Model file for the job. Use its own axes, mm. Face numbers are marked on the shaded views. A direction names the side the tool comes from. Give positions to 0.01 mm unless a question says otherwise; leave off trailing zeros. Write each loop counter-clockwise with the first axis right and the second up, starting at its lowest first coordinate (ties: lowest second). Pieces come first, ordered by that corner, then holes.
```python
from build123d import *

# Parameters (mm, degrees)
F0_W     = 30
F0_H     = 50
F1_DEPTH = 10
F2_R     = 10
F3_DEPTH = 7
F4_R     = 5
F5_R     = 5
F6_R     = 5
F7_R     = 5


with BuildPart() as f1:
    # F0 (on Front) → F1 (new body)
    with BuildSketch(Plane.XZ):
        Rectangle(F0_W, F0_H)
    extrude(amount=-F1_DEPTH)

    # F2 (on face) → F3 (join)
    with BuildSketch(Plane.XZ):
        Circle(F2_R)
    extrude(amount=F3_DEPTH)

    # F4
    f4_edges = [f1.edges().sort_by_distance(p)[0] for p in [
        (15, 5, 25),
    ]]
    fillet(f4_edges, radius=F4_R)

    # F5
    f5_edges = [f1.edges().sort_by_distance(p)[0] for p in [
        (-15, 5, 25),
    ]]
    fillet(f5_edges, radius=F5_R)

    # F6
    f6_edges = [f1.edges().sort_by_distance(p)[0] for p in [
        (15, 5, -25),
    ]]
    fillet(f6_edges, radius=F6_R)

    # F7
    f7_edges = [f1.edges().sort_by_distance(p)[0] for p in [
        (-15, 5, -25),
    ]]
    fillet(f7_edges, radius=F7_R)


solid = f1.part
```
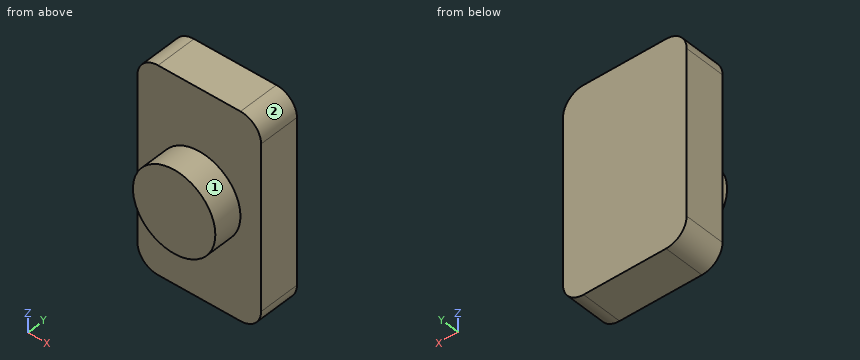
1. Slice it at A-A, the plane x = 0. Write the cut outline in (y, z), and give its area (3 significant figures).
Calculated:
outline: (-7, -10) - (0, -10) - (0, -25) - (10, -25) - (10, 25) - (0, 25) - (0, 10) - (-7, 10) - close
area: 640 mm2
2. Slice it at D-D, the plane x = -10.5. Write the cut outline in (y, z).
Calculated:
outline: (0, -24.97) - (10, -24.97) - (10, 24.97) - (0, 24.97) - close
3. Probe probe 1 along Y at (x, z) = (-9, -23); probe 2 along X at (y, z) = (-4.25, -1.5); probe 3 along Z at (x, y) = (8.75, -1.75). List the from-to ranges inside material, lowest first.
Calculated:
probe 1: y = 0 to 10
probe 2: x = -9.89 to 9.89
probe 3: z = -4.84 to 4.84
4. Slice it at B-B, the plane z = 0. Write the cut outline in (x, y).
Calculated:
outline: (-15, 0) - (-10, 0) - (-10, -7) - (10, -7) - (10, 0) - (15, 0) - (15, 10) - (-15, 10) - close
5. Pin check, flat tips, straight feed: P1, Ø4, axis at x = 10, z = -3.5, coming from the -Y side; P2, Ø1, axis at y = -3.5, z = -11.5, coming from the +X side; P3, Ø1.5, axis at y = -5, z = 7, coming from the +X side. Stop position of each tip, or through.
Calculated:
P1: stops at y = -7
P2: passes through
P3: stops at x = 7.81
6. Which spindle directions (+Z, -Z, +X, -X, +Y, -Y) get a long thin tool onto all of the face, cutting with end or side? Do the marked faces 1 and 2. Say none if no direction does.
Calculated:
face 1: -Y
face 2: +Z, +X, +Y, -Y
7. Slice it at C-C, the plane z = 18.5. Write the cut outline in (x, y), and give its area (3 significant figures).
Calculated:
outline: (-15, 0) - (15, 0) - (15, 10) - (-15, 10) - close
area: 300 mm2
